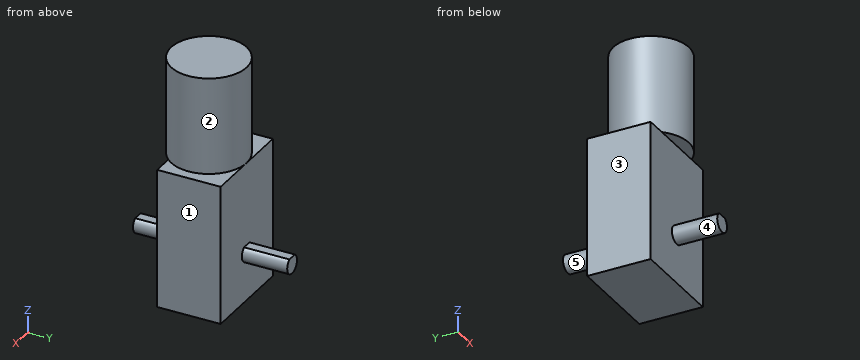
from build123d import *

# Parameters (mm, degrees)
SKETCH190_W             = 46
SKETCH190_H             = 32
PAD124_DEPTH            = 21
SKETCH191_R             = 12.5
PAD125_DEPTH            = 32
PAD126_DEPTH            = 15
PAD127_DEPTH            = 15
BODY099_PITCH_ANGLE     = -90
BODY099_PLACEMENT_ANGLE = 90


with BuildPart() as part:
    # Sketch190 → Pad124 (new body)
    with BuildSketch(Plane.XY):
        with Locations((7, 0)):
            Rectangle(SKETCH190_W, SKETCH190_H)
    extrude(amount=PAD124_DEPTH)

    # Sketch191 (on Face2 of Pad124) → Pad125 (join)
    with BuildSketch(Plane.YZ.offset(30)):
        with Locations((0, 12.5)):
            Circle(SKETCH191_R)
    extrude(amount=PAD125_DEPTH)

    # Sketch192 (on Face4 of Pad125) → Pad126 (join)
    with BuildSketch(Plane(origin=(0, 0, 0), x_dir=(1, 0, 0), z_dir=(0, 0, -1))):
        with BuildLine():
            ThreePointArc((2.5, 1.658312), (-3, 0), (2.5, -1.658312))
            Line((2.5, 1.658312), (2.5, -1.658312))
        make_face()
    extrude(amount=PAD126_DEPTH)

    # Sketch193 (on Face5 of Pad126) → Pad127 (join)
    with BuildSketch(Plane.XY.offset(21)):
        with BuildLine():
            ThreePointArc((2.5, 1.658312), (-3, 0), (2.5, -1.658312))
            Line((2.5, 1.658312), (2.5, -1.658312))
        make_face()
    extrude(amount=PAD127_DEPTH)


with BuildPart() as part_1:
    # Body099 pitch: moved
    add(part.part.rotate(Axis((0, 0, 0), (0, 1, 0)), BODY099_PITCH_ANGLE))


with BuildPart() as part_2:
    # Body099 placement: moved
    add(part_1.part.moved(Location((0, -24, 0))).rotate(Axis((0, -24, 0), (0, 0, 1)), BODY099_PLACEMENT_ANGLE))


solid = part_2.part
Work out the finished part from the listing and answer in its coordinate system (mm). Face numbers are marked on the shaded views. A direction names the side the tool comes from. Give positions to 0.01 mm unless a question says otherwise; leave off trailing zeros. Loops run counter-clockwise (first coordinate to the right, second up) from the corner with the lowest first, then second, coordinate; pieces in that order, holes last. Notation, with made-up numbers: (66, 15) - (97, 15) arc R25 ccw to (97, 32) - close; hole circle Ø4 at (74.5, -8.75). An arc over 180 degrees is marked (long way). Answer in a Markdown table with one row per item.
(1) Flat-ended cylindrical pins translate along their axes: pin 1 Ø3.5 at (x, y) = (-0.5, -52) entering from +Z; pin 2 Ø10 at (x, z) = (8.5, 24) entering from -Y; pin 3 Ø2 at (x, z) = (-7.5, 19) entering from +Y; pin 4 Ø10 at (y, z) = (-18.5, 53) entering from -X. Find the tip coordinate at first contact, or state that the pin passes through.
Results list:
| item | result |
|---|---|
| pin 1 | stops at z = 2.5 |
| pin 2 | stops at y = -45 |
| pin 3 | stops at y = -24 |
| pin 4 | passes through |
(2) A tool of negligible diameter and unlimited length cuts with its end or side. For the marked faces 1, 2, 3, 4 and 5, from which of +Z, -Z, +X, -X, +Y, -Y can it reach the whole face along a straight path? Write none if from no direction.
Results list:
| item | result |
|---|---|
| face 1 | +Z, -Z, +X, +Y, -Y |
| face 2 | +Z |
| face 3 | +Z, -Z, -X, +Y, -Y |
| face 4 | -Y |
| face 5 | +Y |
(3) Section C-C (x = -10.5) is taken. Give the vertices of the cut face in (y, z).
Results list:
| item | result |
|---|---|
| outline | (-45, -16) - (-24, -16) - (-24, 30) - (-29.72, 30) - (-29.72, 62) - (-43.28, 62) - (-43.28, 30) - (-45, 30) - close |
(4) Section A-A (z = 0) is taken. Give the vertices of the cut face in (x, y), and give its area (3 significant figures).
Results list:
| item | result |
|---|---|
| outline | (-16, -45) - (-3, -45) - (-3, -60) - (3, -60) - (3, -45) - (16, -45) - (16, -24) - (3, -24) - (3, -9) - (-3, -9) - (-3, -24) - (-16, -24) - close |
| area | 852 mm² |
(5) Consider L1, parallel to Z at x = 15.5, y = -35.5; L2, parallel to Y at x = 8, z = 6.5; L3, parallel to X at y = -51, z = 0. Determine where each line is inside the solid, lowest interval first. Write a range as [from, to].
Results list:
| item | result |
|---|---|
| L1 | z = [-16, 30] |
| L2 | y = [-45, -24] |
| L3 | x = [-3, 3] |
(6) Section B-B (y = -36.5) is taken. Give the vertices of the cut face in (x, z).
Results list:
| item | result |
|---|---|
| outline | (-16, -16) - (16, -16) - (16, 30) - (12.5, 30) - (12.5, 62) - (-12.5, 62) - (-12.5, 30) - (-16, 30) - close |
(7) Section D-D (z = 28) is taken. Give the vertices of the cut face in (x, y), and give its area (3 significant figures).
Results list:
| item | result |
|---|---|
| outline | (-16, -45) - (16, -45) - (16, -24) - (-16, -24) - close |
| area | 672 mm² |
